Here's how the part is built. I have some questions about the finished solid (model axes, mm). A direction names the side the tool comes from. Give positions to 0.01 mm unless a question says otherwise; leave off trailing zeros. Loops run counter-clockwise (first coordinate to the right, second up) from the corner with the lowest first, then second, coordinate; pieces in that order, holes last.
Q1. We'd pull the mould along X, two halves only. Please class faces 1 (the face through (9.75, 6, -37)), 2 (the face through (54, 10.15, -14)), 3 (the face through (31.75, 6, -14)): +X half, -X half, draft (parallel to the pull), parting line (faces both ways), or undercut.
Q2. If we section it at A-A (y = -1): Please give me the cut outline in (x, z).
Q3. For faces 4 (the face through (38, 10.15, -14)), 5 (the face through (16, 6, -3.925)), 6 (the face through (31.75, 6, -38)), 7 (the face through (38, 6, -48.775)), which set-ups out of +Z, -Z, +X, -X, +Y, -Y let a thin tool reach every point of the face, with its end or its side?
Q4. If we section it at B-B (z = -50.4): Please give me the cut outline in (x, y), plus the area to 3 significant figures.
Q5. If we section it at D-D (z = -8): Please give me the cut outline in (x, y).
Q6. Will these pins go through, and if not, where does the flat tip stop? P1, Ø2.5, axis at x = 9.5, y = 5, coming from the -Z side; P2, Ø7, axis at y = 6.5, z = -18.5, coming from the +X side; P3, Ø4, axis at y = 4, z = -47.5, coming from the +X side; P4, Ø1, axis at x = 8.5, y = -1, coming from the -Z side.
Q7. I need wall thicknesses on line 1 (X direction, y = 8, z = -29.5); line 2 (Z direction, x = 5.5, y = 3.25); line 3 (Z direction, x = 14.9, y = 1.35). Which ranges of each line are inside material? Lowest first, please.
Q8. If we section it at C-C (x = 29.5): Please give me the cut outline in (y, z) (3 decimals), plus the area to 3 significant figures.
from build123d import *

# Parameters (mm, degrees)
SKETCH1_R           = 1.5
BOSS_EXTRUDE1_DEPTH = 1.65
SKETCH2_W           = 14.9
SKETCH2_H           = 2.5
SKETCH2_W_2         = 4.5
SKETCH2_W_3         = 9.5
BOSS_EXTRUDE2_DEPTH = 2.5
SKETCH3_W           = 5
SKETCH3_H           = 15
SKETCH3_W_2         = 10
SKETCH3_H_2         = 10
SKETCH3_W_3         = 2.4
SKETCH3_H_3         = 20.7
SKETCH3_H_4         = 33
BOSS_EXTRUDE3_DEPTH = 8.5
SKETCH4_W           = 10
SKETCH4_H           = 7.75
BOSS_EXTRUDE4_DEPTH = 10
CUT_EXTRUDE1_DEPTH  = 10
SKETCH6_W           = 6
SKETCH6_H           = 6
BOSS_EXTRUDE5_DEPTH = 3.5


with BuildPart() as part:
    # Sketch1 → Boss-Extrude1 (new body)
    with BuildSketch(Plane(origin=(0, 0, 0), x_dir=(1, 0, 0), z_dir=(0, 1, 0))):
        Polygon((68, 5), (65.5, 2.5), (65.5, 0), (0, 0), (0, 52.7), (65.5, 52.7), (65.5, 40.75), (68, 38.25), align=None)
        with Locations((13.75, 50.4)):
            Circle(SKETCH1_R, mode=Mode.SUBTRACT)
        with Locations((14.9, 2.04)):
            Circle(SKETCH1_R, mode=Mode.SUBTRACT)
    extrude(amount=BOSS_EXTRUDE1_DEPTH)

    # Sketch2 → Boss-Extrude2 (add)
    with BuildSketch(Plane(origin=(0, 0, 0), x_dir=(-1, 0, 0), z_dir=(0, -1, 0))):
        with Locations((-57.05, 2)):
            Rectangle(SKETCH2_W, SKETCH2_H)
        with Locations((-62.25, 50.7)):
            Rectangle(SKETCH2_W_2, SKETCH2_H)
        with Locations((-27.25, 50.7)):
            Rectangle(SKETCH2_W_3, SKETCH2_H)
    extrude(amount=BOSS_EXTRUDE2_DEPTH)

    # Sketch3 → Boss-Extrude3 (add)
    with BuildSketch(Plane(origin=(0, 1.65, 0), x_dir=(1, 0, 0), z_dir=(0, 1, 0))):
        with Locations((12.25, 36.7)):
            Rectangle(SKETCH3_W, SKETCH3_H)
        with Locations((7.5, 23.7)):
            Rectangle(SKETCH3_W_2, SKETCH3_H_2)
        with Locations((16.45, 14.275)):
            Rectangle(SKETCH3_W_3, SKETCH3_H_3)
        with Locations((29.3, 14.275)):
            Rectangle(SKETCH3_W_3, SKETCH3_H_3)
        with Locations((37.7, 14.275)):
            Rectangle(SKETCH3_W_3, SKETCH3_H_3)
        with Locations((50.55, 14.275)):
            Rectangle(SKETCH3_W_3, SKETCH3_H_3)
        with Locations((16.45, 38.425)):
            Rectangle(SKETCH3_W_3, SKETCH3_H_3)
        with Locations((29.3, 38.425)):
            Rectangle(SKETCH3_W_3, SKETCH3_H_3)
        with Locations((37.7, 38.425)):
            Rectangle(SKETCH3_W_3, SKETCH3_H_3)
        with Locations((50.55, 38.425)):
            Rectangle(SKETCH3_W_3, SKETCH3_H_3)
        with Locations((61, 42.95)):
            Rectangle(SKETCH3_W, SKETCH3_H_2)
        with Locations((64.5, 21)):
            Rectangle(SKETCH3_W, SKETCH3_H_4)
        with Locations((32.95, 14.275)):
            Rectangle(SKETCH3_W_3, SKETCH3_H_2)
        with Locations((32.95, 38.425)):
            Rectangle(SKETCH3_W_3, SKETCH3_H_2)
        with Locations((54.2, 38.425)):
            Rectangle(SKETCH3_W_3, SKETCH3_H_2)
        with Locations((54.2, 14.275)):
            Rectangle(SKETCH3_W_3, SKETCH3_H_2)
    extrude(amount=BOSS_EXTRUDE3_DEPTH)

    # Sketch4 → Boss-Extrude4 (add)
    with BuildSketch(Plane(origin=(0, 1.65, 0), x_dir=(1, 0, 0), z_dir=(0, 1, 0))):
        with Locations((6, 13.625)):
            Rectangle(SKETCH4_W, SKETCH4_H)
    extrude(amount=BOSS_EXTRUDE4_DEPTH)

    # Sketch5 → Cut-Extrude1 (cut)
    with BuildSketch(Plane.ZY.offset(-1)):
        Polygon((-17.5, 8.15), (-15.5, 11.65), (-17.5, 11.65), align=None)
        Polygon((-9.75, 11.65), (-9.75, 8.15), (-10.75, 11.65), align=None)
    extrude(amount=-CUT_EXTRUDE1_DEPTH, mode=Mode.SUBTRACT)

    # Sketch6 → Boss-Extrude5 (add)
    with BuildSketch(Plane(origin=(0, 1.65, 0), x_dir=(1, 0, 0), z_dir=(0, 1, 0))):
        with Locations((5, 48.7)):
            Rectangle(SKETCH6_W, SKETCH6_H)
    extrude(amount=BOSS_EXTRUDE5_DEPTH)


solid = part.part
Check sheet entries:
1. face 1: -X half
1. face 2: draft
1. face 3: undercut
2. outline: (22.5, -51.95) - (32, -51.95) - (32, -49.45) - (22.5, -49.45) - close; (49.6, -3.25) - (64.5, -3.25) - (64.5, -0.75) - (49.6, -0.75) - close; (60, -51.95) - (64.5, -51.95) - (64.5, -49.45) - (60, -49.45) - close
3. face 4: +Z, -Z, +X, +Y
3. face 5: +Z, +X, -X, +Y
3. face 6: +Z, -Z, +Y
3. face 7: -Z, +X, +Y
4. outline: (0, 0) - (12.25, 0) - (12.25, 1.65) - (8, 1.65) - (8, 5.15) - (2, 5.15) - (2, 1.65) - (0, 1.65) - close; (15.25, 0) - (22.5, 0) - (22.5, -2.5) - (32, -2.5) - (32, 0) - (60, 0) - (60, -2.5) - (64.5, -2.5) - (64.5, 0) - (65.5, 0) - (65.5, 1.65) - (15.25, 1.65) - close
4. area: 159 mm2
5. outline: (0, 0) - (68, 0) - (68, 1.65) - (67, 1.65) - (67, 10.15) - (62, 10.15) - (62, 1.65) - (51.75, 1.65) - (51.75, 10.15) - (49.35, 10.15) - (49.35, 1.65) - (38.9, 1.65) - (38.9, 10.15) - (36.5, 10.15) - (36.5, 1.65) - (30.5, 1.65) - (30.5, 10.15) - (28.1, 10.15) - (28.1, 1.65) - (17.65, 1.65) - (17.65, 10.15) - (15.25, 10.15) - (15.25, 1.65) - (0, 1.65) - close
6. P1: stops at z = -44.2
6. P2: stops at x = 67
6. P3: stops at x = 63.5
6. P4: passes through
7. line 1: x = 9.75 to 14.75, 15.25 to 17.65, 28.1 to 30.5, 36.5 to 38.9, 49.35 to 51.75, 62 to 67
7. line 2: z = -51.7 to -45.7, -28.7 to -18.7, -17.5 to -9.75
7. line 3: z = -52.7 to -51.36, -49.44 to -3.54, -0.54 to 0
8. outline: (-2.5, -51.95) - (0, -51.95) - (0, -52.7) - (1.65, -52.7) - (1.65, -48.775) - (10.15, -48.775) - (10.15, -28.075) - (1.65, -28.075) - (1.65, -24.625) - (10.15, -24.625) - (10.15, -3.925) - (1.65, -3.925) - (1.65, 0) - (0, 0) - (0, -49.45) - (-2.5, -49.45) - close
8. area: 445 mm2
